Design review of the part built by this model. Coordinates are the model's own, in mm. Round coordinates to 2 decimals unless told otherwise and drop trailing zeros. Loops run counter-clockwise (first coordinate to the right, second up) from the corner with the lowest first, then second, coordinate; pieces in that order, holes last. Notation, with made-up numbers: M 51.5,-31 L 81.5,-31 A29 cw 81.5,-8 Z; hole C 29,28.25 d8. An arc over 180 degrees is marked long. Use a Markdown table: item, result.
from build123d import *
from build123d.topology import SkipClean

# Parameters (mm, degrees)
SKETCH1_R           = 6
SKETCH1_R_2         = 8
BOSS_EXTRUDE1_DEPTH = 3
BOSS_EXTRUDE2_START = -2
SKETCH1_3_R         = 6
BOSS_EXTRUDE2_DEPTH = 2
SKETCH6_R           = 4.1
CUT_EXTRUDE1_DEPTH  = 3


with BuildPart() as part:
    # Sketch1 → Boss-Extrude1 (new body)
    with BuildSketch(Plane.XY):
        with BuildLine():
            ThreePointArc((12.899477, 38.647167), (5.904038, 33.483464), (1.096566, 40.728338))
            Line((1.096566, 40.728338), (-7.799149, 1.781371))
            ThreePointArc((-7.799149, 1.781371), (0.896329, 7.949629), (8, 0))
            ThreePointArc((8, 0), (7.984502, -0.497727), (7.938067, -0.993525))
            Line((7.938067, -0.993525), (12.899477, 38.647167))
        make_face()
        with Locations((6.945927, 39.39231)):
            Circle(SKETCH1_R)
        Circle(SKETCH1_R_2)
    extrude(amount=BOSS_EXTRUDE1_DEPTH)

    # Sketch1<3> → Boss-Extrude2 (add)
    with BuildSketch(Plane.XY.offset(BOSS_EXTRUDE2_START)):
        with Locations(Location((6.945927, 39.39231, 0), (0, 0, 167.134016))):
            Circle(SKETCH1_3_R)
    extrude(amount=BOSS_EXTRUDE2_DEPTH)

    # Sketch3 → Cut-Revolve1 (revolve, cut)
    with SkipClean():  # the faces are left unmerged after this step: merging them gives an invalid solid
        with BuildSketch(Plane(origin=(6.945927, 0, 0), x_dir=(0, 0, -1), z_dir=(1, 0, 0))):
            with BuildLine():
                ThreePointArc((9, 39.39231), (7.828427, 42.220737), (5, 43.39231))
                Line((5, 43.39231), (5, 35.39231))
                ThreePointArc((5, 35.39231), (7.828427, 36.563883), (9, 39.39231))
            make_face()
            with BuildLine():
                Line((5, 35.39231), (5, 43.39231))
                ThreePointArc((5, 43.39231), (1, 39.39231), (5, 35.39231))
            make_face()
        revolve(axis=Axis((6.945927, 43.39231, -5), (0, -1, 0)), mode=Mode.SUBTRACT)

    # Chamfer1: read off the stored shape, not the designer's step
    # Chamfer1 outline → Chamfer1 (revolve, cut)
    with SkipClean():  # the faces are left unmerged after this step: merging them gives an invalid solid
        with BuildSketch(Plane(origin=(6.945927, 39.39231, 0), x_dir=(1, 0, 0), z_dir=(0, -1, 0))):
            Polygon((2.601903, -1.961892), (2.601903, -2), (6, -2), (6, 0), align=None)
        revolve(axis=Axis((6.945927, 39.39231, 0), (0, 0, 1)), mode=Mode.SUBTRACT)

    # Sketch6 → Cut-Extrude1 (cut)
    with SkipClean():  # the faces are left unmerged after this step: merging them gives an invalid solid
        with BuildSketch(Plane(origin=(0, 0, 0), x_dir=(-1, 0, 0), z_dir=(0, 0, -1))):
            Circle(SKETCH6_R)
        extrude(amount=-CUT_EXTRUDE1_DEPTH, mode=Mode.SUBTRACT)


solid = part.part
1. Wall thickness on line 1 along Z through (x, y) = (-2.25, 18.5); line 2 along Y through (x, z) = (2.5, 2.75); line 3 along X through (y, z) = (17, 0.7): over which ranges is each line inside the solid? List them lowest first. Write a range as from..to.
Check values:
| item | result |
|---|---|
| line 1 | z = 0..3 |
| line 2 | y = -7.6..-3.25, 3.25..43.42 |
| line 3 | x = -4.32..10.19 |
2. The part is to be moulded in two halves that separate along Y. For faces 1 (the face through (0.534, 4.065, 1.479)), 2 (the face through (9.502, 38.333, -1.867)), 3 (the face through (2, 19, 3)), say which applies: pulls with the +Y half, pulls with the -Y half, needs draft (parallel to the pull), parting line crosses it, or undercut.
Check values:
| item | result |
|---|---|
| face 1 | undercut |
| face 2 | parting line crosses it |
| face 3 | needs draft |
3. Take a section at C-C on y = 13.5. Give the boundary of the cut face in (x, z).
Check values:
| item | result |
|---|---|
| outline | M -5.12,0 L 9.75,0 L 9.75,3 L -5.12,3 Z |
4. Take a section at B-B on x = 0. Give the boundary of the cut face in (y, z).
Check values:
| item | result |
|---|---|
| outline | M -8,0 L -4.1,0 L -4.1,3 L -8,3 Z; M 4.1,0 L 35.93,0 L 35.93,3 L 4.1,3 Z |
5. Take a section at D-D on x = -5. Give the boundary of the cut face in (y, z) (3 decimals).
Check values:
| item | result |
|---|---|
| outline | M -6.245,0 L 14.037,0 L 14.037,3 L -6.245,3 Z |
6. Take a section at A-A on y = 3.5. Give the boundary of the cut face in (x, z), and give its area (3 significant figures).
Check values:
| item | result |
|---|---|
| outline | M -7.41,0 L -2.14,0 L -2.14,3 L -7.41,3 Z; M 2.14,0 L 8.5,0 L 8.5,3 L 2.14,3 Z |
| area | 34.9 mm² |
7. Insertion check: pin 1 (10.5 mm diameter, centred on x = -2.5, y = 26.5, fed in from -Z); pin 2 (6 mm diameter, centred on x = 10.5, y = 32.5, fed in from -Z). Each pin has a flat end and moves straight along its axis. Give the tip position at first contact, or say it passes through.
Check values:
| item | result |
|---|---|
| pin 1 | stops at z = 0 |
| pin 2 | stops at z = -0.72 |
